For this review, take the finished solid that the model builds, in its own axes (mm). Coordinates: 2 decimals unless noted, no trailing zeros. Write each loop counter-clockwise with the first axis right and the second up, starting at its lowest first coordinate (ties: lowest second). Pieces come first, ordered by that corner, then holes.
1) We need section A-A on z = 5. Write out the cut boundary in (x, y).
2) We need section C-C on y = -25.5. Write out the cut boundary in (x, z), then the cut area to 3 significant figures.
3) We need section B-B on x = -25. Write out the cut boundary in (y, z), then the cut area to 3 significant figures.
4) Insertion check: P1, Ø5, axis at x = 0, y = 60, coming from the -Z side; P2, Ø1, axis at y = -50.5, z = 4, coming from the -X side; P3, Ø2, axis at x = -20, z = 5, coming from the -Y side. Each pin has a flat end and moves straight along its axis. Give the tip position at first contact, or say it passes through.
5) We need section D-D on y = 53.5. Write out the cut boundary in (x, z), then the cut area to 3 significant figures.
6) To check wall thickness, follow line 1 along Y through (x, z) = (3, 0.5); line 2 along Y through (x, z) = (-25, 2.75); line 3 along Z through (x, y) = (-2, 61). State the ranges of each line that lie inside material, in increasing order.
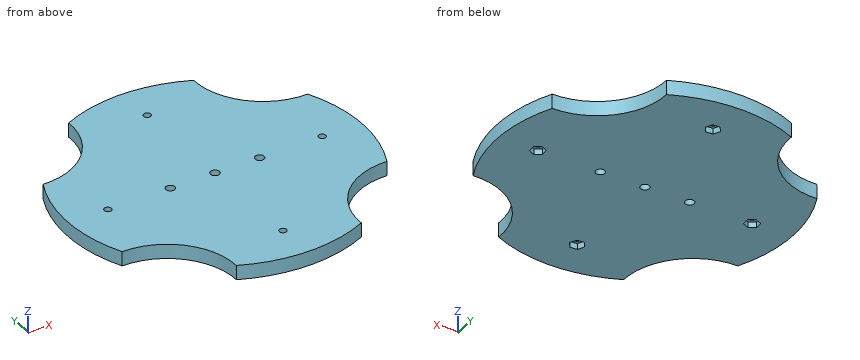
from build123d import *

# Parameters (mm, degrees)
SKETCH1_R           = 82
BOSS_EXTRUDE1_DEPTH = 8
SKETCH2_R           = 2
CUT_EXTRUDE1_DEPTH  = 15
CIRPATTERN2_COUNT   = 4
CUT_EXTRUDE3_DEPTH  = 3.2
CIRPATTERN3_COUNT   = 4
SKETCH10_R          = 2.5
CUT_EXTRUDE4_DEPTH  = 10
CUT_EXTRUDE5_START  = -10
CUT_EXTRUDE5_DEPTH  = 10
CIRPATTERN4_COUNT   = 4


with BuildPart() as part:
    # Sketch1 → Boss-Extrude1 (new body)
    with BuildSketch(Plane.XY):
        Circle(SKETCH1_R)
    extrude(amount=BOSS_EXTRUDE1_DEPTH)

    # Sketch2 → Cut-Extrude1 (cut)
    with BuildSketch(Plane.XY.offset(8)):
        with Locations((0, 60)):
            Circle(SKETCH2_R)
    cut_extrude1 = extrude(amount=-CUT_EXTRUDE1_DEPTH, mode=Mode.SUBTRACT)

    # CirPattern2: Cut-Extrude1 ×4 about axis
    cirpattern2_axis = Axis((0, 0, 0), (0, 0, 1))
    for i in range(1, CIRPATTERN2_COUNT):
        add(cut_extrude1.rotate(cirpattern2_axis, i * 360 / CIRPATTERN2_COUNT), mode=Mode.SUBTRACT)

    # Sketch7 → Cut-Extrude3 (cut)
    with BuildSketch(Plane(origin=(0, 0, 0), x_dir=(-1, 0, 0), z_dir=(0, 0, -1))):
        Polygon((1.788462671, 63.624187441), (-2.244407056, 63.360947827), (-4.032869728, 59.736760386), (-1.788462671, 56.375812559), (2.244407056, 56.639052173), (4.032869728, 60.263239614), align=None)
    cut_extrude3 = extrude(amount=-CUT_EXTRUDE3_DEPTH, mode=Mode.SUBTRACT)

    # CirPattern3: Cut-Extrude3 ×4 about axis
    cirpattern3_axis = Axis((0, 0, 0), (0, 0, 1))
    for i in range(1, CIRPATTERN3_COUNT):
        add(cut_extrude3.rotate(cirpattern3_axis, i * 360 / CIRPATTERN3_COUNT), mode=Mode.SUBTRACT)

    # Sketch10 → Cut-Extrude4 (cut)
    with BuildSketch(Plane.XY.offset(8)):
        Circle(SKETCH10_R)
        with Locations((25, 0)):
            Circle(SKETCH10_R)
        with Locations((-25, 0)):
            Circle(SKETCH10_R)
    extrude(amount=-CUT_EXTRUDE4_DEPTH, mode=Mode.SUBTRACT)

    # Sketch11 → Cut-Extrude5 (cut)
    with BuildSketch(Plane.XY.offset(8).offset(CUT_EXTRUDE5_START)):
        with BuildLine():
            ThreePointArc((-35.000836658, 74.154847672), (-46.112698372, 46.112698372), (-74.154847672, 35.000836658))
            ThreePointArc((-74.154847672, 35.000836658), (-57.982756057, 57.982756057), (-35.000836658, 74.154847672))
        make_face()
    cut_extrude5 = extrude(amount=CUT_EXTRUDE5_DEPTH, mode=Mode.SUBTRACT)

    # CirPattern4: Cut-Extrude5 ×4 about axis
    cirpattern4_axis = Axis((0, 0, 0), (0, 0, 1))
    for i in range(1, CIRPATTERN4_COUNT):
        add(cut_extrude5.rotate(cirpattern4_axis, i * 360 / CIRPATTERN4_COUNT), mode=Mode.SUBTRACT)


solid = part.part
Result:
1. outline: (-74.15, -35) arc R38 cw to (-35, -74.15) arc R82 ccw to (35, -74.15) arc R38 cw to (74.15, -35) arc R82 ccw to (74.15, 35) arc R38 cw to (35, 74.15) arc R82 ccw to (-35, 74.15) arc R38 cw to (-74.15, 35) arc R82 ccw to start; hole circle Ø4 at (-60, 0); hole circle Ø5 at (-25, 0); hole circle Ø5 at (0, 0); hole circle Ø4 at (0, -60); hole circle Ø4 at (0, 60); hole circle Ø5 at (25, 0); hole circle Ø4 at (60, 0)
2. outline: (-77.93, 0) - (77.93, 0) - (77.93, 8) - (-77.93, 8) - close
2. area: 1,250 mm2
3. outline: (-78.1, 0) - (-2.5, 0) - (-2.5, 8) - (-78.1, 8) - close; (2.5, 0) - (78.1, 0) - (78.1, 8) - (2.5, 8) - close
3. area: 1,210 mm2
4. P1: stops at z = 3.2
4. P2: stops at x = -42.72
4. P3: stops at y = -79.77
5. outline: (-40.36, 0) - (40.36, 0) - (40.36, 8) - (-40.36, 8) - close
5. area: 646 mm2
6. line 1: y = -81.95 to -61.81, -58.17 to 58.19, 61.83 to 81.95
6. line 2: y = -78.1 to -2.5, 2.5 to 78.1
6. line 3: z = 3.2 to 8
